Could you check a few things on this model? Use its own coordinates, in mm. A direction names the side the tool comes from. Round coordinates to 2 decimals unless told otherwise and drop trailing zeros. Loops run counter-clockwise (first coordinate to the right, second up) from the corner with the lowest first, then second, coordinate; pieces in that order, holes last. Notation, with made-up numbers: (83.5, -23) - (139.5, -23) arc R11 cw to (139.5, -19) - close; hole circle Ø8 at (87, -39.5). An arc over 180 degrees is marked (long way). Use one line per item in the form item = value.
```python
from build123d import *

# Parameters (mm, degrees)
SKETCH1_W           = 63.5
SKETCH1_H           = 63.5
BOSS_EXTRUDE1_DEPTH = 63.5
SKETCH2_RX          = 2.667
SKETCH2_RY          = 1.9685
CUT_EXTRUDE1_DEPTH  = 3.175
SKETCH3_W           = 57.15
SKETCH3_H           = 57.15
CUT_EXTRUDE2_DEPTH  = 53.975
CUT_EXTRUDE3_REACH  = 79.771
SKETCH4_R           = 4.064
CUT_EXTRUDE4_REACH  = 79.771
SKETCH5_R           = 3.175


with BuildPart() as part:
    # Sketch1 → Boss-Extrude1 (new body)
    with BuildSketch(Plane.XY):
        Rectangle(SKETCH1_W, SKETCH1_H)
    extrude(amount=BOSS_EXTRUDE1_DEPTH)

    # Sketch2 → Cut-Extrude1 (cut)
    with BuildSketch(Plane.XY.offset(63.5)):
        with Locations((0, 0)):
            Ellipse(SKETCH2_RX, SKETCH2_RY)
        with Locations((20, 0)):
            Ellipse(SKETCH2_RX, SKETCH2_RY)
        with Locations((-20, 0)):
            Ellipse(SKETCH2_RX, SKETCH2_RY)
    extrude(amount=-CUT_EXTRUDE1_DEPTH, mode=Mode.SUBTRACT)

    # Sketch3 → Cut-Extrude2 (cut)
    with BuildSketch(Plane(origin=(0, 31.75, 0), x_dir=(1, 0, 0), z_dir=(0, 1, 0))):
        with Locations((0, -31.75)):
            Rectangle(SKETCH3_W, SKETCH3_H)
    extrude(amount=-CUT_EXTRUDE2_DEPTH, mode=Mode.SUBTRACT)

    # Sketch4 → Cut-Extrude3 (cut, up to next)
    with BuildSketch(Plane(origin=(0, 0, 0), x_dir=(-1, 0, 0), z_dir=(0, 0, -1)), mode=Mode.PRIVATE) as cut_extrude3_sk1:
        with Locations((-12.5984, -12.7)):
            Circle(SKETCH4_R)
    cut_extrude3_tool1 = extrude(cut_extrude3_sk1.sketch, amount=-CUT_EXTRUDE3_REACH, mode=Mode.PRIVATE) & part.part
    # Sketch4 → Cut-Extrude3 (cut, up to next)
    with BuildSketch(Plane(origin=(0, 0, 0), x_dir=(-1, 0, 0), z_dir=(0, 0, -1)), mode=Mode.PRIVATE) as cut_extrude3_sk2:
        with Locations((12.7, -12.7)):
            Circle(SKETCH4_R)
    cut_extrude3_tool2 = extrude(cut_extrude3_sk2.sketch, amount=-CUT_EXTRUDE3_REACH, mode=Mode.PRIVATE) & part.part
    add(cut_extrude3_tool1.solids().sort_by_distance((12.5984, -12.7, 0))[0], mode=Mode.SUBTRACT)
    add(cut_extrude3_tool2.solids().sort_by_distance((-12.7, -12.7, 0))[0], mode=Mode.SUBTRACT)

    # Sketch5 → Cut-Extrude4 (cut, up to next)
    with BuildSketch(Plane(origin=(0, 0, 0), x_dir=(-1, 0, 0), z_dir=(0, 0, -1)), mode=Mode.PRIVATE) as cut_extrude4_sk1:
        with Locations((-19.05, 12.7)):
            Circle(SKETCH5_R)
    cut_extrude4_tool1 = extrude(cut_extrude4_sk1.sketch, amount=-CUT_EXTRUDE4_REACH, mode=Mode.PRIVATE) & part.part
    # Sketch5 → Cut-Extrude4 (cut, up to next)
    with BuildSketch(Plane(origin=(0, 0, 0), x_dir=(-1, 0, 0), z_dir=(0, 0, -1)), mode=Mode.PRIVATE) as cut_extrude4_sk2:
        with Locations((0, 12.7)):
            Circle(SKETCH5_R)
    cut_extrude4_tool2 = extrude(cut_extrude4_sk2.sketch, amount=-CUT_EXTRUDE4_REACH, mode=Mode.PRIVATE) & part.part
    # Sketch5 → Cut-Extrude4 (cut, up to next)
    with BuildSketch(Plane(origin=(0, 0, 0), x_dir=(-1, 0, 0), z_dir=(0, 0, -1)), mode=Mode.PRIVATE) as cut_extrude4_sk3:
        with Locations((19.05, 12.7)):
            Circle(SKETCH5_R)
    cut_extrude4_tool3 = extrude(cut_extrude4_sk3.sketch, amount=-CUT_EXTRUDE4_REACH, mode=Mode.PRIVATE) & part.part
    add(cut_extrude4_tool1.solids().sort_by_distance((19.05, 12.7, 0))[0], mode=Mode.SUBTRACT)
    add(cut_extrude4_tool2.solids().sort_by_distance((0, 12.7, 0))[0], mode=Mode.SUBTRACT)
    add(cut_extrude4_tool3.solids().sort_by_distance((-19.05, 12.7, 0))[0], mode=Mode.SUBTRACT)


solid = part.part
```
1. For P1, Ø7.5, axis at x = 0, y = 12.7, coming from the -Z side; P2, Ø5, axis at x = 19.05, y = 12.7, coming from the -Z side (3 decimals), each with a flat end and sliding along its axis, tell me the tip position at first contact or that it passes through.
Solution:
P1 = 0
P2 = 60.325
2. On a 3-axis mill with a long thin cutter (end or side, diameter ignored), from which of +Z, -Z, +X, -X, +Y, -Y can I reach the whole of each face in a straight line? I mean faces 5 (the face through (0, 0, 0)), 6 (the face through (15.8, -15.2, 1.6)), 7 (the face through (28.575, 5, 32)). Say none if no direction works.
Solution:
face_5 = -Z, +X, -X, +Y, -Y
face_6 = -Z
face_7 = +Y
3. If we section it at B-B, the plane y = -12.7: Write out the boundary of the cut face in (x, z) (3 decimals).
Solution:
outline = (-31.75, 0) - (-16.764, 0) - (-16.764, 3.175) - (-28.575, 3.175) - (-28.575, 60.325) - (28.575, 60.325) - (28.575, 3.175) - (16.662, 3.175) - (16.662, 0) - (31.75, 0) - (31.75, 63.5) - (-31.75, 63.5) - close; (-8.636, 0) - (8.534, 0) - (8.534, 3.175) - (-8.636, 3.175) - close
4. If we section it at C-C, the plane y = 12.7: Write out the boundary of the cut face in (x, z) (3 decimals), plus the area to 3 significant figures.
Solution:
outline = (-31.75, 0) - (-22.225, 0) - (-22.225, 3.175) - (-28.575, 3.175) - (-28.575, 60.325) - (28.575, 60.325) - (28.575, 3.175) - (22.225, 3.175) - (22.225, 0) - (31.75, 0) - (31.75, 63.5) - (-31.75, 63.5) - close; (-15.875, 0) - (-3.175, 0) - (-3.175, 3.175) - (-15.875, 3.175) - close; (3.175, 0) - (15.875, 0) - (15.875, 3.175) - (3.175, 3.175) - close
area = 706 mm^2
5. If we section it at D-D, the plane x = 0: Count the separate pieces of the cut face and the enclosed holes in it, plus the area to 3 significant figures.
Solution:
separate_pieces = 3
enclosed_holes = 0
area = 915 mm^2
6. We'd pull the mould along X, two halves only. Please class faces 1 (the face through (-1.5, 9.9, 1.6)), 2 (the face through (0, 5, 60.325)), 3 (the face through (31.75, 0, 31)), 4 (the face through (-31.75, 0, 31)): +X half, -X half, draft (parallel to the pull), parting line (faces both ways), or undercut.
Solution:
face_1 = undercut
face_2 = undercut
face_3 = +X half
face_4 = -X half
7. Please list where these lines run through material, in increasing order: line 1 along Z through (x, y) = (6, 26.5) (3 decimals); line 2 along Y through (x, z) = (-19, 1); line 3 along X through (y, z) = (12, 1).
Solution:
line_1 = 0 to 3.175, 60.325 to 63.5
line_2 = -31.75 to 9.53, 15.87 to 31.75
line_3 = -31.75 to -22.15, -15.95 to -3.1, 3.1 to 15.95, 22.15 to 31.75
8. If we section it at A-A, the plane x = -12.7: Write out the boundary of the cut face in (y, z) (3 decimals).
Solution:
outline = (-31.75, 0) - (-16.764, 0) - (-16.764, 3.175) - (-22.225, 3.175) - (-22.225, 60.325) - (31.75, 60.325) - (31.75, 63.5) - (-31.75, 63.5) - close; (-8.636, 0) - (31.75, 0) - (31.75, 3.175) - (-8.636, 3.175) - close
